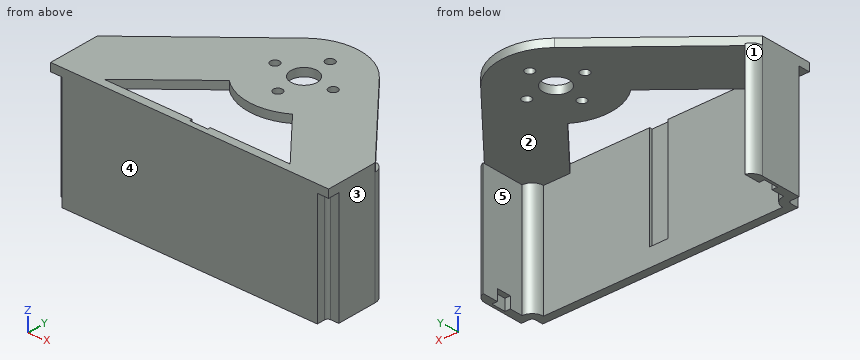
from build123d import *

# Parameters (mm, degrees)
SKETCH_R        = 1
SKETCH_R_2      = 2.9
PAD_DEPTH       = 1.8
PAD001_DEPTH    = 25
SKETCH004_W     = 4
SKETCH004_H     = 0.6
POCKET_DEPTH    = 22.8
SKETCH005_W     = 1.2
SKETCH005_H     = 3.2
POCKET001_DEPTH = 2.5


with BuildPart() as part:
    # Sketch → Pad (new body)
    with BuildSketch(Plane.XY):
        with BuildLine():
            Line((9.431274, 8.050532), (27.4, -13))
            Line((27.4, -13), (27.4, -24.5))
            Line((27.4, -24.5), (-34.1, -24.5))
            Line((-34.1, -24.5), (-34.1, -13))
            Line((-8.091275, 9.396344), (-34.1, -13))
            ThreePointArc((9.431274, 8.050532), (0.94958, 12.363588), (-8.091275, 9.396344))
        make_face()
        with Locations((6.45, 0)):
            Circle(SKETCH_R, mode=Mode.SUBTRACT)
        with Locations((-6.45, 0)):
            Circle(SKETCH_R, mode=Mode.SUBTRACT)
        with Locations((0, 6.45)):
            Circle(SKETCH_R, mode=Mode.SUBTRACT)
        with Locations((0, -6.45)):
            Circle(SKETCH_R, mode=Mode.SUBTRACT)
        Circle(SKETCH_R_2, mode=Mode.SUBTRACT)
        with BuildLine():
            Line((-8.273758, -9.236066), (-23.909335, -22.7))
            Line((-23.909335, -22.7), (17.273072, -22.7))
            Line((17.273072, -22.7), (6.766294, -10.391211))
            ThreePointArc((-8.273758, -9.236066), (-0.94958, -12.363588), (6.766294, -10.391211))
        make_face(mode=Mode.SUBTRACT)
    extrude(amount=PAD_DEPTH)

    # Sketch001 → Pad001 (new body)
    with BuildSketch(Plane(origin=(0, 0, 0), x_dir=(1, 0, 0), z_dir=(0, 0, -1))):
        with BuildLine():
            Line((24.9, 24.5), (-31.6, 24.5))
            Line((-31.6, 24.5), (-31.6, 22.7))
            ThreePointArc((-32.3, 22), (-31.805025, 22.205025), (-31.6, 22.7))
            Line((-32.3, 22), (-34.1, 22))
            Line((-34.1, 22), (-34.1, 13))
            ThreePointArc((-34.1, 13), (-33.6, 11.5), (-32.3, 10.6))
            Line((-32.3, 10.6), (-32.3, 20.2))
            ThreePointArc((-32.3, 20.2), (-30.532233, 20.932233), (-29.8, 22.7))
            Line((-29.8, 22.7), (23.1, 22.7))
            ThreePointArc((23.1, 22.7), (23.832233, 20.932233), (25.6, 20.2))
            Line((25.6, 10.6), (25.6, 20.2))
            ThreePointArc((25.6, 10.6), (26.9, 11.5), (27.4, 13))
            Line((27.4, 22), (27.4, 13))
            Line((25.6, 22), (27.4, 22))
            ThreePointArc((24.9, 22.7), (25.105025, 22.205025), (25.6, 22))
            Line((24.9, 24.5), (24.9, 22.7))
        make_face()
    extrude(amount=PAD001_DEPTH)

    # Sketch004 → Pocket (cut)
    with BuildSketch(Plane.XY.offset(1.8)):
        with Locations((-2.4, -23)):
            Rectangle(SKETCH004_W, SKETCH004_H)
    extrude(amount=-POCKET_DEPTH, mode=Mode.SUBTRACT)

    # Sketch005 → Pocket001 (cut)
    with BuildSketch(Plane(origin=(0, 0, -25), x_dir=(1, 0, 0), z_dir=(0, 0, -1))):
        with Locations((26.2, 15.7)):
            Rectangle(SKETCH005_W, SKETCH005_H)
        with Locations((-32.9, 15.7)):
            Rectangle(SKETCH005_W, SKETCH005_H)
    extrude(amount=-POCKET001_DEPTH, mode=Mode.SUBTRACT)


solid = part.part
Source: CAD feature listing. Evaluate the final solid. Frame: model axes, mm. Face numbers are marked on the shaded views. A direction names the side the tool comes from. Round coordinates to 2 decimals unless told otherwise and drop trailing zeros. Loops run counter-clockwise (first coordinate to the right, second up) from the corner with the lowest first, then second, coordinate; pieces in that order, holes last. Notation, with made-up numbers: M 42.25,-4 L 54.25,-4 A26 cw 54.25,22 Z; hole C 79.5,-20 d3. An arc over 180 degrees is marked long. Return JSON: item names as keys, results as strings. Group by question number.
1. Section query C-C on z = -4. Output: boundary loops of the cut face in (x, y).
2. Section query B-B on x = -6.45. Output: boundary loops of the cut face in (y, z), and give its area (3 significant figures).
3. Section query D-D on x = 4. Output: boundary loops of the cut face in (y, z), and give its area (3 significant figures).
4. Material intervals for line 1 along Y through (x, z) = (0, 0.5); line 2 along Y through (x, z) = (-27, -1.75); line 3 along Z through (x, y) = (-1.5, 6), sorted ascending. Write a range as from..to.
5. Reachability of the marked faces 1 and 2 from +Z, -Z, +X, -X, +Y, -Y: full face, straight path, thin tool, end or side. Return the list, or none.
6. Section query A-A on y = -6.45. Output: boundary loops of the cut face in (x, z).
7. Mould query, pull axis X, two halves, no side actions, for the marked faces 3, 4 and 5. Classes: released by +X, released by -X, zero draft, split by the parting line, or undercut.
8. Pin query (flat end, axial travel): pin 1 (6.5 mm diameter, centred on x = 0, y = 0, fed in from -Z); pin 2 (0.9 mm diameter, centred on x = 26, z = -9.5, fed in from -Y); pin 3 (1.3 mm diameter, centred on x = 26, y = -15.5, fed in from -Z); pin 4 (1 mm diameter, centred on x = -10, y = -13, fed in from -Z). Return the tip coordinate at first contact, or that it passes through.
Checks:
{
 "1": {"outline": "M -34.1,-22 L -32.3,-22 A0.7 cw -31.6,-22.7 L -31.6,-24.5 L 24.9,-24.5 L 24.9,-22.7 A0.7 cw 25.6,-22 L 27.4,-22 L 27.4,-13 A2.5 ccw 25.6,-10.6 L 25.6,-20.2 A2.5 ccw 23.1,-22.7 L -0.4,-22.7 L -0.4,-23.3 L -4.4,-23.3 L -4.4,-22.7 L -29.8,-22.7 A2.5 ccw -32.3,-20.2 L -32.3,-10.6 A2.5 ccw -34.1,-13 Z"},
 "2": {"outline": "M -24.5,-25 L -22.7,-25 L -22.7,1.8 L -24.5,1.8 Z; M -10.59,0 L -1,0 L -1,1.8 L -10.59,1.8 Z; M 1,0 L 10.59,0 L 10.59,1.8 L 1,1.8 Z", "area": "82.8 mm²"},
 "3": {"outline": "M -24.5,-25 L -22.7,-25 L -22.7,1.8 L -24.5,1.8 Z; M -11.74,0 L 11.74,0 L 11.74,1.8 L -11.74,1.8 Z", "area": "90.5 mm²"},
 "4": {"line 1": "y = -24.5..-22.7, -12.4..-7.45, -5.45..-2.9, 2.9..5.45, 7.45..12.4", "line 2": "y = -24.5..-22.7", "line 3": "z = 0..1.8"},
 "5": {"face 1": "+Z, -Z, -X, +Y", "face 2": "-Z, +Y"},
 "6": {"outline": "M -26.49,0 L -1,0 L -1,1.8 L -26.49,1.8 Z; M 1,0 L 21.81,0 L 21.81,1.8 L 1,1.8 Z"},
 "7": {"face 3": "released by +X", "face 4": "zero draft", "face 5": "undercut"},
 "8": {"pin 1": "stops at z = 0", "pin 2": "stops at y = -22", "pin 3": "stops at z = -22.5", "pin 4": "passes through"}
}
